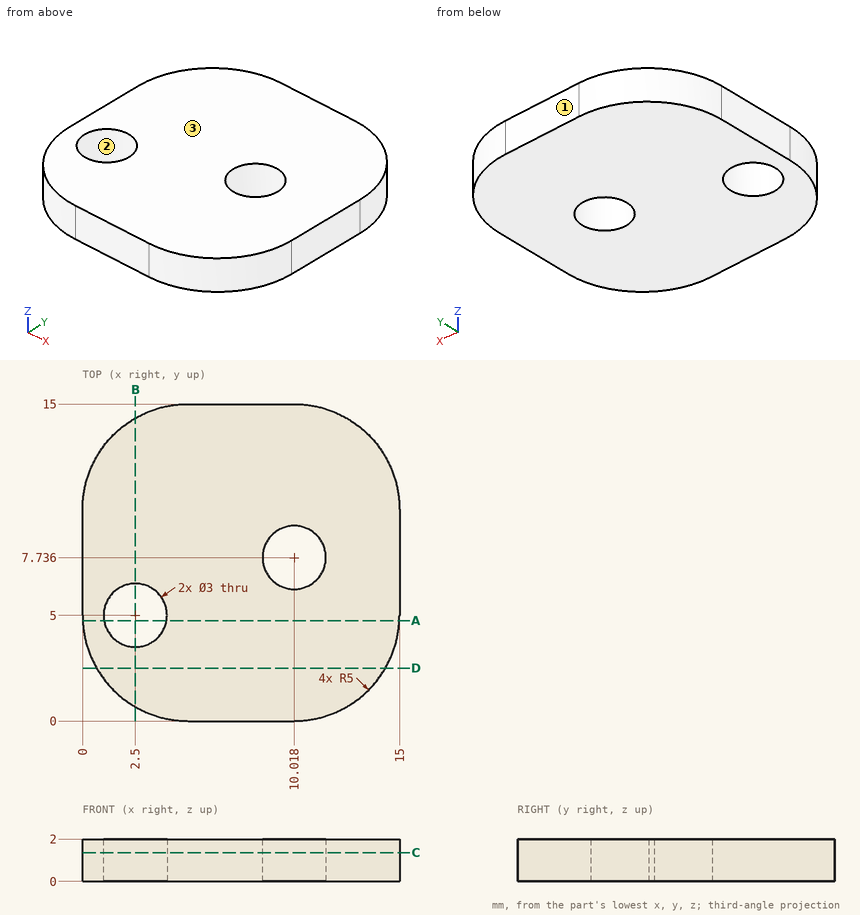
Part print with two shaded views. Sizes in mm from the minimum x, y, z corner. Coordinates: 2 decimals unless noted, no trailing zeros. Order: outer loops, then holes, each group sorted by start corner. A loop starts at its lowest first (then second) coordinate and runs counter-clockwise, first axis right, second up.
(1) Pin check, flat tips, straight feed: pin 1 Ø8 at (x, y) = (4, 12.5) entering from -Z; pin 2 Ø2.5 at (x, y) = (10.02, 7.74) entering from -Z. Stop position of each tip, or through.
Solution:
pin 1: stops at z = 0
pin 2: passes through
(2) Mould opens along Y. For the marked faces 1, 2 and 3 say: released by +Y, released by -Y, zero draft, split by the parting line, or undercut.
Solution:
face 1: released by +Y
face 2: undercut
face 3: zero draft
(3) Saw through at C-C, the plane z = 1.35. Write the cut outline in (x, y), and give its area (3 significant figures).
Solution:
outline: (0, 5) arc R5 ccw to (5, 0) - (10, 0) arc R5 ccw to (15, 5) - (15, 10) arc R5 ccw to (10, 15) - (5, 15) arc R5 ccw to (0, 10) - close; hole circle Ø3 at (2.5, 5); hole circle Ø3 at (10.02, 7.74)
area: 189 mm2
(4) Drill centre lines: L1, parallel to X at y = 8, z = 1.3 (1 decimal); L2, parallel to Y at x = 3, z = 1.1 (1 decimal); L3, parallel to Y at x = 10.75, z = 0.55 (1 decimal). Where is each one in solid material? Low to high.
Solution:
L1: x = 0 to 8.5, 11.5 to 15
L2: y = 0.4 to 3.6, 6.4 to 14.6
L3: y = 0.1 to 6.4, 9 to 14.9
(5) Saw through at A-A, the plane y = 4.75. Write the cut outline in (x, z).
Solution:
outline: (0.01, 0) - (1.02, 0) - (1.02, 2) - (0.01, 2) - close; (3.98, 0) - (14.99, 0) - (14.99, 2) - (3.98, 2) - close
(6) Saw through at D-D, the plane y = 2.5. Write the cut outline in (x, z).
Solution:
outline: (0.67, 0) - (14.33, 0) - (14.33, 2) - (0.67, 2) - close
(7) Saw through at B-B, the plane x = 2.5. Write the cut outline in (y, z).
Solution:
outline: (0.67, 0) - (3.5, 0) - (3.5, 2) - (0.67, 2) - close; (6.5, 0) - (14.33, 0) - (14.33, 2) - (6.5, 2) - close
